Verification items for this drawing (mm, ordinates from the low corner). Coordinates: 2 decimals unless noted, no trailing zeros. Order: outer loops, then holes, each group sorted by start corner. A loop starts at its lowest first (then second) coordinate and runs counter-clockwise, first axis right, second up. Notation, with made-up numbers: M 53,13.5 L 62,13.5 A33 ccw 62,49.5 Z; hole C 6.25,84.5 d11. An arc over 180 degrees is marked long. Answer as a JSON object with one key per item and string values. Group by question number.
(1) Cross-section at A-A (z = 1.25). Enter the section's corners in (x, y).
(2) Cross-section at B-B (x = 63). Enter the section's corners in (y, z), plus the area to 3 significant figures.
(3) Gauge pin test, flat ends, axial feed: pin 1 Ø1 at (y, z) = (32.5, 1) entering from +X; pin 2 Ø0.6 at (y, z) = (1, 1.5) entering from +X; pin 3 Ø8 at (x, y) = (99.5, 29) entering from -Z; pin 4 Ø1 at (x, z) = (59, 1.5) entering from -Y. Record the tip position at first contact, or that the pin passes through.
(4) Material ranges on line 1 (Y direction, x = 65, z = 1.85); line 2 (Y direction, x = 113.5, z = 1); line 3 (X direction, y = 5, z = 1.85), recorded low to high.
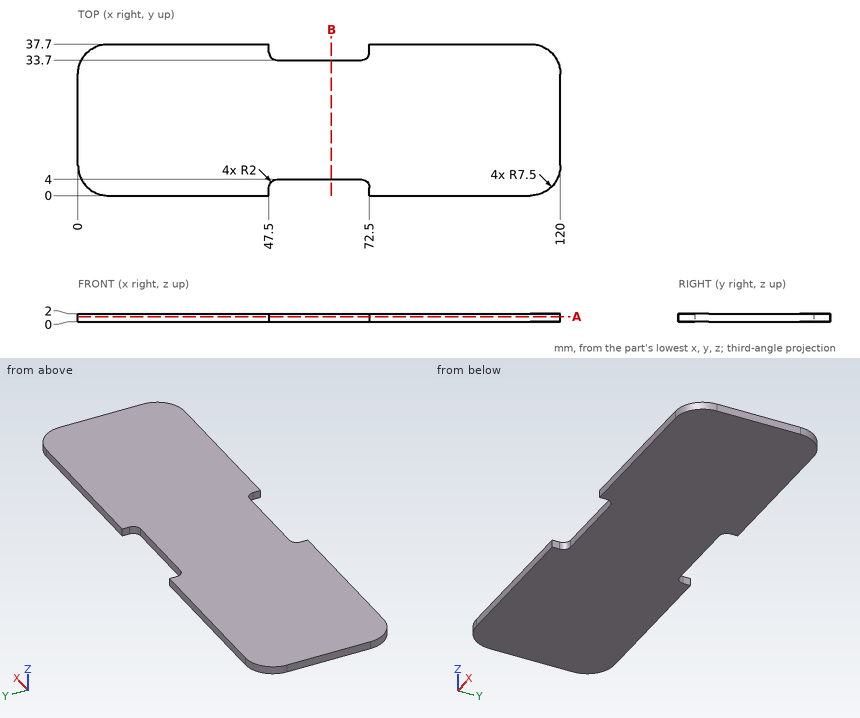
Taken from the geometry:
{
 "1": {"outline": "M 0,7.5 A7.5 ccw 7.5,0 L 47.5,0 L 47.5,2 A2 cw 49.5,4 L 70.5,4 A2 cw 72.5,2 L 72.5,0 L 112.5,0 A7.5 ccw 120,7.5 L 120,30.2 A7.5 ccw 112.5,37.7 L 72.5,37.7 L 72.5,35.7 A2 cw 70.5,33.7 L 49.5,33.7 A2 cw 47.5,35.7 L 47.5,37.7 L 7.5,37.7 A7.5 ccw 0,30.2 Z"},
 "2": {"outline": "M 4,0 L 33.7,0 L 33.7,2 L 4,2 Z", "area": "59.4 mm²"},
 "3": {"pin 1": "stops at x = 119.78", "pin 2": "stops at x = 116.72", "pin 3": "stops at z = 0", "pin 4": "stops at y = 4"},
 "4": {"line 1": "y = 4 to 33.7", "line 2": "y = 0.07 to 37.63", "line 3": "x = 0.43 to 119.57"}
}
